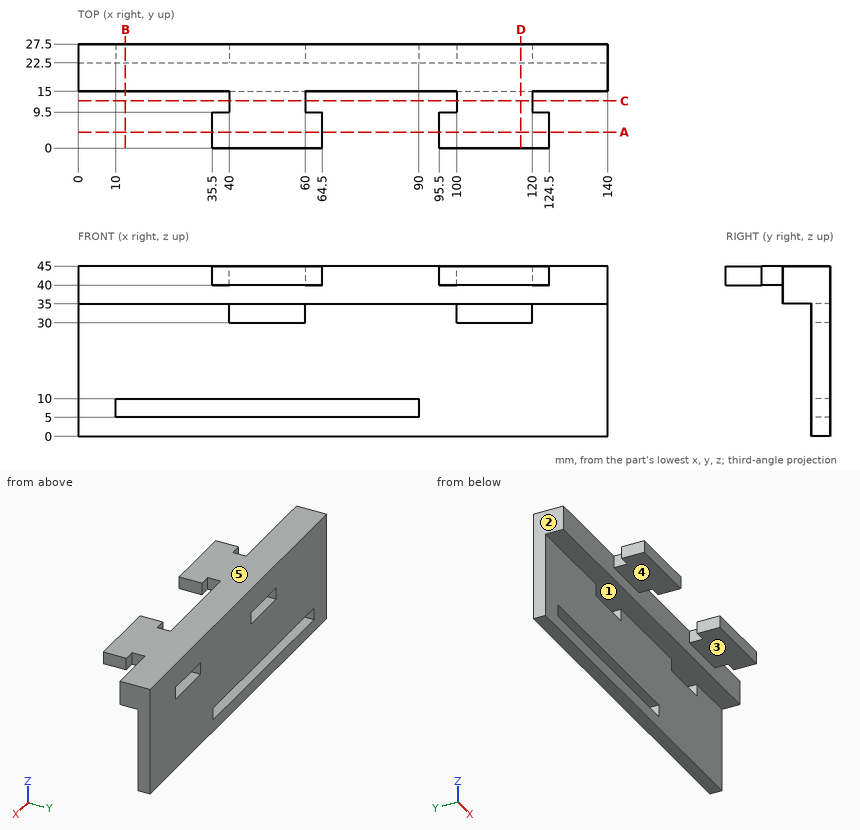
The drawing under review shows one solid part. Ordinate dimensions are in mm from its lowest x, y, z. A direction names the side the tool comes from. Round coordinates to 2 decimals unless told otherwise and drop trailing zeros. Loops run counter-clockwise (first coordinate to the right, second up) from the corner with the lowest first, then second, coordinate; pieces in that order, holes last. Notation, with made-up numbers: (-15.75, -33) -> (41.25, -33) arc R22 cw to (41.25, -24) -> close; hole circle Ø8 at (1, 51). An arc over 180 degrees is marked (long way). Answer in a Markdown table with one row per item.
1) Consider section C-C, the plane y = 12.5. Write out the cut boundary in (x, z), plus the area to 3 significant figures.
Taken from the geometry:
| item | result |
|---|---|
| outline | (40, 40) -> (60, 40) -> (60, 45) -> (40, 45) -> close; (100, 40) -> (120, 40) -> (120, 45) -> (100, 45) -> close |
| area | 200 mm² |
2) For pin 1 Ø5 at (x, y) = (86.5, 10.5) entering from -Z; pin 2 Ø2.5 at (y, z) = (6.5, 43) entering from -X; pin 3 Ø1 at (x, y) = (50.5, 15) entering from -Z; pin 4 Ø4 at (x, z) = (75, 32) entering from -Y, all flat-tipped, find the tip position at first contact; note any pin that passes through.
Taken from the geometry:
| item | result |
|---|---|
| pin 1 | passes through |
| pin 2 | stops at x = 35.5 |
| pin 3 | stops at z = 35 |
| pin 4 | stops at y = 22.5 |
3) Draft analysis for pull direction Z (two halves, no side actions). For the marked faces 1, 2 and 3, state which applies: pulls with the +Z half, pulls with the -Z half, needs draft (parallel to the pull), parting line crosses it, or undercut.
Taken from the geometry:
| item | result |
|---|---|
| face 1 | undercut |
| face 2 | needs draft |
| face 3 | pulls with the -Z half |
4) Wall thickness on line 1 along Z through (x, y) = (83, 22.75); line 2 along X through (y, z) = (10.5, 43); line 3 along Y through (x, z) = (24, 28): over which ranges is each line inside the solid? List them lowest first.
Taken from the geometry:
| item | result |
|---|---|
| line 1 | z = 0 to 5, 10 to 45 |
| line 2 | x = 40 to 60, 100 to 120 |
| line 3 | y = 22.5 to 27.5 |
5) Consider section D-D, the plane x = 117. Write out the cut boundary in (y, z), plus the area to 3 significant figures.
Taken from the geometry:
| item | result |
|---|---|
| outline | (0, 40) -> (15, 40) -> (15, 35) -> (27.5, 35) -> (27.5, 45) -> (0, 45) -> close; (22.5, 0) -> (27.5, 0) -> (27.5, 30) -> (22.5, 30) -> close |
| area | 350 mm² |
6) Tool access review of the marked faces 4 and 5: name each direction out of +Z, -Z, +X, -X, +Y, -Y from which nothing blocks a thin tool from reaching the whole face with its end or side.
Taken from the geometry:
| item | result |
|---|---|
| face 4 | -Z, +X, -X, -Y |
| face 5 | +Z, +X, -X, +Y, -Y |
7) Consider section A-A, the plane y = 4.25. Write out the cut boundary in (x, z), plus the area to 3 significant figures.
Taken from the geometry:
| item | result |
|---|---|
| outline | (35.5, 40) -> (64.5, 40) -> (64.5, 45) -> (35.5, 45) -> close; (95.5, 40) -> (124.5, 40) -> (124.5, 45) -> (95.5, 45) -> close |
| area | 290 mm² |
8) Consider section B-B, the plane x = 12.5. Write out the cut boundary in (y, z), plus the area to 3 significant figures.
Taken from the geometry:
| item | result |
|---|---|
| outline | (15, 35) -> (22.5, 35) -> (22.5, 10) -> (27.5, 10) -> (27.5, 45) -> (15, 45) -> close; (22.5, 0) -> (27.5, 0) -> (27.5, 5) -> (22.5, 5) -> close |
| area | 275 mm² |
